Geometry check sheet. Reference: the model listing, model coordinates, mm. A direction names the side the tool comes from. Coordinates: 2 decimals unless noted, no trailing zeros. Loops run counter-clockwise (first coordinate to the right, second up) from the corner with the lowest first, then second, coordinate; pieces in that order, holes last.
from build123d import *

# Parameters (mm, degrees)
SKETCH1_W           = 254
SKETCH1_H           = 254
BOSS_EXTRUDE1_DEPTH = 533.4
SKETCH2_R           = 25
BOSS_EXTRUDE2_DEPTH = 50
SKETCH3_W           = 1046.8
SKETCH3_H           = 267.639830062
CUT_EXTRUDE1_DEPTH  = 254


with BuildPart() as part:
    # Sketch1 → Boss-Extrude1 (new, symmetric)
    with BuildSketch(Plane.XY):
        Rectangle(SKETCH1_W, SKETCH1_H)
    extrude(amount=BOSS_EXTRUDE1_DEPTH, both=True)

    # Sketch2 → Boss-Extrude2 (add)
    with BuildSketch(Plane.XY.offset(533.4)):
        with Locations(Location((0, 0, 0), (0, 0, 180))):
            Circle(SKETCH2_R)
    boss_extrude2 = extrude(amount=BOSS_EXTRUDE2_DEPTH)

    # Mirror1: Boss-Extrude2 across plane
    add(boss_extrude2.mirror(Plane.XY))

    # Sketch3 → Cut-Extrude1 (cut)
    with BuildSketch(Plane(origin=(127, 0, 0), x_dir=(0, 0, -1), z_dir=(1, 0, 0))):
        with Locations((0, -46.819915031)):
            Rectangle(SKETCH3_W, SKETCH3_H)
    extrude(amount=-CUT_EXTRUDE1_DEPTH, mode=Mode.SUBTRACT)


solid = part.part
(1) Sectioned sample at D-D on z = 183.5. Record the cut outline in (x, y), and give its area (3 significant figures).
Findings:
outline: (-127, 87) - (127, 87) - (127, 127) - (-127, 127) - close
area: 10,200 mm2
(2) Sectioned sample at A-A on y = 67.5. Record the cut outline in (x, z).
Findings:
outline: (-127, -533.4) - (127, -533.4) - (127, -523.4) - (-127, -523.4) - close; (-127, 523.4) - (127, 523.4) - (127, 533.4) - (-127, 533.4) - close
(3) Sectioned sample at B-B on x = 0. Record the cut outline in (y, z), and give its area (3 significant figures).
Findings:
outline: (-127, -533.4) - (-25, -533.4) - (-25, -583.4) - (25, -583.4) - (25, -533.4) - (127, -533.4) - (127, 533.4) - (25, 533.4) - (25, 583.4) - (-25, 583.4) - (-25, 533.4) - (-127, 533.4) - (-127, 523.4) - (87, 523.4) - (87, -523.4) - (-127, -523.4) - close
area: 52,000 mm2
(4) Sectioned sample at C-C on y = 0. Record the cut outline in (x, z).
Findings:
outline: (-127, -533.4) - (-25, -533.4) - (-25, -583.4) - (25, -583.4) - (25, -533.4) - (127, -533.4) - (127, -523.4) - (-127, -523.4) - close; (-127, 523.4) - (127, 523.4) - (127, 533.4) - (25, 533.4) - (25, 583.4) - (-25, 583.4) - (-25, 533.4) - (-127, 533.4) - close
(5) Scan lines: L1, parallel to Z at x = -27.5, y = -52; L2, parallel to Z at x = -14.5, y = -10.5; L3, parallel to Y at x = -94, z = -383. Record each from-to range of solid material in increasing order.
Findings:
L1: z = -533.4 to -523.4, 523.4 to 533.4
L2: z = -583.4 to -523.4, 523.4 to 583.4
L3: y = 87 to 127
(6) Gauge pin test, flat ends, axial feed: pin 1 Ø4 at (x, y) = (-99, 75.5) entering from -Z; pin 2 Ø12 at (x, z) = (94, 464.5) entering from -Y; pin 3 Ø12 at (x, y) = (-67.5, -68) entering from +Z. Record the tip position at first contact, or that the pin passes through.
Findings:
pin 1: stops at z = -533.4
pin 2: stops at y = 87
pin 3: stops at z = 533.4
(7) Access from +Z, -Z, +X, -X, +Y, -Y to the whole of each face (thin tool, end or side, straight path). Record for faces 1 (the flat face through (2, -21, 523.4)), 2 (the cylindrical face through (-23.846, -7.509, -558.05)), 3 (the flat face through (0, 0, -583.4)), 4 (the cylindrical face through (-23.846, -7.509, 558.05)).
Findings:
face 1: +X, -X, -Y
face 2: -Z
face 3: -Z, +X, -X, +Y, -Y
face 4: +Z
(8) Draft check along Z on faces 5 (the flat face through (2, 87, 7)), 6 (the flat face through (0, 0, 583.4)), 7 (the flat face through (-2, 127, 7)). Enter one of: +Z half, -Z half, draft (parallel to the pull), parting line (faces both ways), or undercut.
Findings:
face 5: undercut
face 6: +Z half
face 7: draft
